Here's how the part is built. I have some questions about the finished solid (model axes, mm). Face numbers are marked on the shaded views. Give positions to 0.01 mm unless a question says otherwise; leave off trailing zeros. Loops run counter-clockwise (first coordinate to the right, second up) from the corner with the lowest first, then second, coordinate; pieces in that order, holes last. Notation, with made-up numbers: (83, -19) - (132, -19) arc R25 cw to (132, 18) - close; hole circle Ø7 at (33, 55.25). An arc over 180 degrees is marked (long way). Return JSON: item names as keys, results as strings. Group by question number.
(1) For P1, Ø1, axis at x = 8.5, z = 1, coming from the +Y side; P2, Ø1.5, axis at x = 15.5, z = 0.5, coming from the +Y side; P3, Ø2, axis at x = 6, y = -1, coming from the +Z side, each with a flat end and sliding along its axis, tell me the tip position at first contact or that it passes through.
(2) I need wall thicknesses on probe 1 along X at (y, z) = (0.8, 0.85); probe 2 along X at (y, z) = (-1.6, -0.05); probe 3 along Z at (x, y) = (3.25, -0.6). Which ranges of each line are inside material? Lowest first, please. Write a range as [from, to].
(3) If we section it at A-A (x = 7.75): Please give me the cut outline in (y, z), then the cut area to 3 significant figures.
(4) If we mould it in two halves opening along Z, with no side actions, what happens to the marked faces 1, 2, 3 and 4? For each: released by +Z, released by -Z, zero draft, split by the parting line, or undercut.
```python
from build123d import *

# Parameters (mm, degrees)
HEX_DIE_START = 1e-06
SKETCH2_R     = 1.866050808
HEX_DIE_DEPTH = 1.599999
SKETCH4_R     = 1.4
INDENT_DEPTH  = 0.2


with BuildPart() as part:
    # BodySke → Base-Revolve (revolve)
    with BuildSketch(Plane.XY):
        Polygon((1.6, 1), (1.6, 1.847575058), (0.142937526, 1.847575058), (0, 1.6), (0, 0), (21.6, 0), (21.6, 1), align=None)
    revolve(axis=Axis((-25.4, 0, 0), (1, 0, 0)))

    # Sketch2 → Hex-Die (cut)
    with BuildSketch(Plane(origin=(0, 0, 0), x_dir=(0, 0, -1), z_dir=(1, 0, 0)).offset(HEX_DIE_START)):
        Circle(SKETCH2_R)
        Polygon((-1.6, 0.923760435), (0, 1.847520869), (1.6, 0.923760435), (1.6, -0.923760435), (0, -1.847520869), (-1.6, -0.923760435), align=None, mode=Mode.SUBTRACT)
    extrude(amount=HEX_DIE_DEPTH, mode=Mode.SUBTRACT)

    # Sketch4 → Indent (cut)
    with BuildSketch(Plane(origin=(0, 0, 0), x_dir=(0, 0, -1), z_dir=(1, 0, 0))):
        Circle(SKETCH4_R)
    extrude(amount=INDENT_DEPTH, mode=Mode.SUBTRACT)


solid = part.part
```
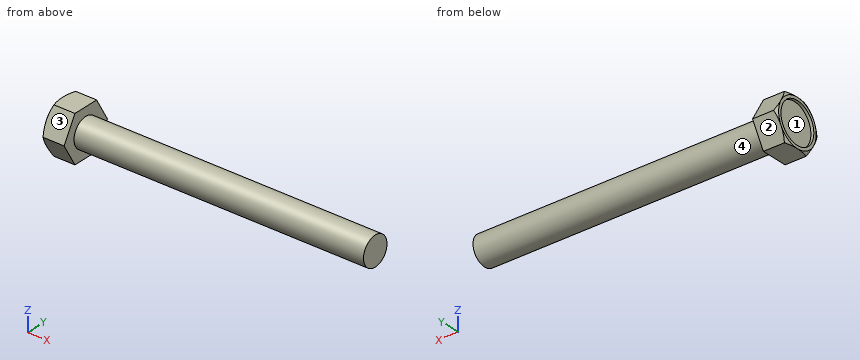
Values:
{
 "1": {"P1": "y = 0.87", "P2": "y = 1", "P3": "z = 1"},
 "2": {"probe 1": "[0.2, 1.6]", "probe 2": "[0, 1.6]", "probe 3": "[-0.8, 0.8]"},
 "3": {"outline": "circle Ø2 at (0, 0)", "area": "3.14 mm2"},
 "4": {"face 1": "undercut", "face 2": "released by -Z", "face 3": "released by +Z", "face 4": "split by the parting line"}
}
